from build123d import *

# Parameters (mm, degrees)
SKETCH_2_R          = 11.5
CUT_EXTRUDE_1_DEPTH = 526.105703645
SKETCH_3_W          = 599
SKETCH_3_H          = 8
CUT_EXTRUDE_2_DEPTH = 10


with BuildPart() as part:
    # Эскиз1 → Повернуть1 (revolve)
    with BuildSketch(Plane.XY, mode=Mode.PRIVATE) as revolve_1_sk:
        Polygon((-300, 50), (-331.5, 50), (-331.5, 44), (-370, 44), (-370, 0), (0, 0), (0, 40), (-300, 40), align=None)
    revolve(revolve_1_sk.sketch.rotate(Axis((0, 0, 0), (0, 1, 0)), 270), axis=Axis((0, 0, 0), (0, 1, 0)))

    # Эскиз2 → Вырез-Вытянуть1 (cut, through all)
    with BuildSketch(Plane(origin=(0, 44, 0), x_dir=(1, 0, 0), z_dir=(0, 1, 0))):
        with Locations(Location((0, 350, 0), (0, 0, 270))):
            Circle(SKETCH_2_R)
        with Locations(Location((77.882326885, 341.224769264, 0), (0, 0, 270))):
            Circle(SKETCH_2_R)
        with Locations(Location((151.859308691, 315.339103766, 0), (0, 0, 270))):
            Circle(SKETCH_2_R)
        with Locations(Location((218.221430651, 273.641018864, 0), (0, 0, 270))):
            Circle(SKETCH_2_R)
        with Locations(Location((273.641018864, 218.221430651, 0), (0, 0, 270))):
            Circle(SKETCH_2_R)
        with Locations(Location((315.339103766, 151.859308691, 0), (0, 0, 270))):
            Circle(SKETCH_2_R)
        with Locations(Location((341.224769264, 77.882326885, 0), (0, 0, 270))):
            Circle(SKETCH_2_R)
        with Locations(Location((350, 0, 0), (0, 0, 270))):
            Circle(SKETCH_2_R)
        with Locations(Location((341.224769264, -77.882326885, 0), (0, 0, 270))):
            Circle(SKETCH_2_R)
        with Locations(Location((315.339103766, -151.859308691, 0), (0, 0, 270))):
            Circle(SKETCH_2_R)
        with Locations(Location((273.641018864, -218.221430651, 0), (0, 0, 270))):
            Circle(SKETCH_2_R)
        with Locations(Location((218.221430651, -273.641018864, 0), (0, 0, 270))):
            Circle(SKETCH_2_R)
        with Locations(Location((151.859308691, -315.339103766, 0), (0, 0, 270))):
            Circle(SKETCH_2_R)
        with Locations(Location((77.882326885, -341.224769264, 0), (0, 0, 270))):
            Circle(SKETCH_2_R)
        with Locations(Location((0, -350, 0), (0, 0, 270))):
            Circle(SKETCH_2_R)
        with Locations(Location((-77.882326885, -341.224769264, 0), (0, 0, 270))):
            Circle(SKETCH_2_R)
        with Locations(Location((-151.859308691, -315.339103766, 0), (0, 0, 270))):
            Circle(SKETCH_2_R)
        with Locations(Location((-218.221430651, -273.641018864, 0), (0, 0, 270))):
            Circle(SKETCH_2_R)
        with Locations(Location((-273.641018864, -218.221430651, 0), (0, 0, 270))):
            Circle(SKETCH_2_R)
        with Locations(Location((-315.339103766, -151.859308691, 0), (0, 0, 270))):
            Circle(SKETCH_2_R)
        with Locations(Location((-341.224769264, -77.882326885, 0), (0, 0, 270))):
            Circle(SKETCH_2_R)
        with Locations(Location((-350, 0, 0), (0, 0, 270))):
            Circle(SKETCH_2_R)
        with Locations(Location((-341.224769264, 77.882326885, 0), (0, 0, 270))):
            Circle(SKETCH_2_R)
        with Locations(Location((-315.339103766, 151.859308691, 0), (0, 0, 270))):
            Circle(SKETCH_2_R)
        with Locations(Location((-273.641018864, 218.221430651, 0), (0, 0, 270))):
            Circle(SKETCH_2_R)
        with Locations(Location((-218.221430651, 273.641018864, 0), (0, 0, 270))):
            Circle(SKETCH_2_R)
        with Locations(Location((-151.859308691, 315.339103766, 0), (0, 0, 270))):
            Circle(SKETCH_2_R)
        with Locations(Location((-77.882326885, 341.224769264, 0), (0, 0, 270))):
            Circle(SKETCH_2_R)
    extrude(amount=-CUT_EXTRUDE_1_DEPTH, mode=Mode.SUBTRACT)

    # Эскиз3 → Вырез-Вытянуть2 (cut)
    with BuildSketch(Plane(origin=(0, 40, 0), x_dir=(1, 0, 0), z_dir=(0, 1, 0))):
        Rectangle(SKETCH_3_W, SKETCH_3_H)
    extrude(amount=-CUT_EXTRUDE_2_DEPTH, mode=Mode.SUBTRACT)


solid = part.part
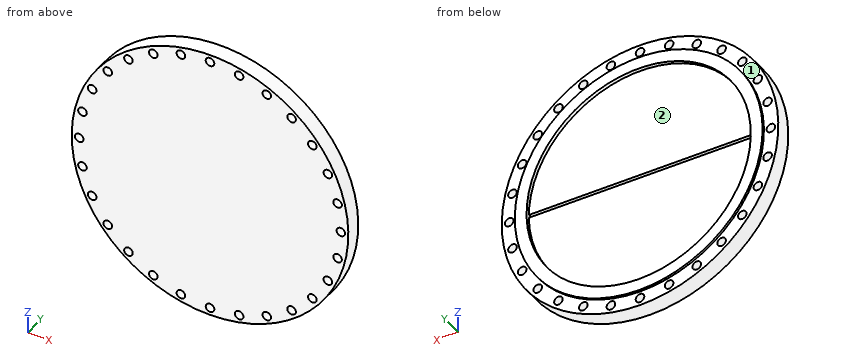
Input: part model. Units: mm. Frame: model coordinates. Face numbers are marked on the shaded views. Coordinates: 2 decimals unless noted, no trailing zeros. Loops run counter-clockwise (first coordinate to the right, second up) from the corner with the lowest first, then second, coordinate; pieces in that order, holes last. Notation, with made-up numbers: (56, 83) -> (92, 83) arc R12 cw to (92, 97) -> close; hole circle Ø6 at (6.5, -29.5). An arc over 180 degrees is marked (long way). Write each question's results on one line, items separated by ' | '. Start each with the question number.
Q1. Pull-direction query (Z, two-part tool) for the marked faces 1 and 2; classes: released by +Z, released by -Z, zero draft, split by the parting line, or undercut.
Q2. Ray query, line 1 (X direction, y = 24, z = -316.5); line 2 (Z direction, x = -87.5, y = 7); line 3 (Z direction, x = 86.5, y = 33). Return the intervals inside material, ascending. Write a range as from..to.
Q3. Section D-D, the plane x = 128.5. Return the cut outline in (y, z), plus the area to 3 significant figures.
Q4. Section C-C, the plane z = 246.5. Return the cut outline in (x, y), plus the area to 3 significant figures.
Q5. Section A-A, the plane x = 0. Return the cut outline in (y, z), plus the area to 3 significant figures.
Q6. Pin query (flat end, axial travel): pin 1 (11 mm diameter, centred on x = 37, y = 37, fed in from -Z); pin 2 (2 mm diameter, centred on x = 79.5, y = 18, fed in from -Z); pin 3 (2 mm diameter, centred on x = 104.5, z = -84.5, fed in from -Y); pin 4 (20.5 mm diameter, centred on x = -77.88, z = -341.22, fed in from +Y). Return the tip coordinate at first contact, or that it passes through.
Q7. Section B-B, the plane y = 8. State how many separate pieces and enclosed holes the cut face has, plus the area to 3 significant figures.
Found:
1) face 1: zero draft | face 2: undercut
2) line 1: -191.64..-163.3, -140.42..140.42, 163.3..191.64 | line 2: -359.5..-347.53, -334.92..334.92, 347.53..359.5 | line 3: -359.75..-348.84, -333.61..-4, 4..333.61, 348.84..359.75
3) outline: (0, -346.97) -> (44, -346.97) -> (44, -305.58) -> (50, -305.58) -> (50, -271.09) -> (40, -271.09) -> (40, -4) -> (30, -4) -> (30, 4) -> (40, 4) -> (40, 271.09) -> (50, 271.09) -> (50, 305.58) -> (44, 305.58) -> (44, 346.97) -> (0, 346.97) -> close | area: 28,700 mm2
4) outline: (-275.93, 0) -> (275.93, 0) -> (275.93, 44) -> (221.65, 44) -> (221.65, 50) -> (170.99, 50) -> (170.99, 40) -> (-170.99, 40) -> (-170.99, 50) -> (-221.65, 50) -> (-221.65, 44) -> (-275.93, 44) -> close | area: 23,500 mm2
5) outline: (0, -370) -> (44, -370) -> (44, -361.5) -> (0, -361.5) -> close; (0, -338.5) -> (44, -338.5) -> (44, -331.5) -> (50, -331.5) -> (50, -300) -> (40, -300) -> (40, -4) -> (30, -4) -> (30, 4) -> (40, 4) -> (40, 300) -> (50, 300) -> (50, 331.5) -> (44, 331.5) -> (44, 338.5) -> (0, 338.5) -> close; (0, 361.5) -> (44, 361.5) -> (44, 370) -> (0, 370) -> close | area: 28,400 mm2
6) pin 1: z = -368.66 | pin 2: z = -361.58 | pin 3: y = 0 | pin 4: through
7) separate pieces: 1 | enclosed holes: 28 | area: 418,000 mm2
